```python
from build123d import *

# Parameters (mm, degrees)
SKETCH1_W           = 120
SKETCH1_H           = 150
SKETCH1_W_2         = 30
SKETCH1_H_2         = 50
BOSS_EXTRUDE1_DEPTH = 5


with BuildPart() as part:
    # Sketch1 → Boss-Extrude1 (new body)
    with BuildSketch(Plane.XY):
        Rectangle(SKETCH1_W, SKETCH1_H)
        with Locations((0, 35)):
            Rectangle(SKETCH1_W_2, SKETCH1_H_2, mode=Mode.SUBTRACT)
    extrude(amount=-BOSS_EXTRUDE1_DEPTH)


solid = part.part
```
Build history of the part. All positions in model axes, mm. A direction names the side the tool comes from. Give positions to 0.01 mm unless a question says otherwise; leave off trailing zeros. Loops run counter-clockwise (first coordinate to the right, second up) from the corner with the lowest first, then second, coordinate; pieces in that order, holes last.
1) Two-plate mould, pull along X, no slides. Class faces 1 (the face through (-1, 1, -5)), 2 (the face through (60, -1, -2)), 3 (the face through (-15, 35, -2)): released by +X, released by -X, zero draft, split by the parting line, or undercut.
Values follow:
face 1: zero draft
face 2: released by +X
face 3: undercut
2) Probe line 1 along X through (y, z) = (10.5, -0.4); line 2 along Y through (x, z) = (-10.5, -3.8). List the from-to ranges inside material, lowest first.
Values follow:
line 1: x = -60 to -15, 15 to 60
line 2: y = -75 to 10, 60 to 75
3) 3-axis set-ups, long thin cutter, end or side, ignore diameter. For faces 4 (the face through (-1, 1, 0)), 5 (the face through (0, 60, -2)): which of +Z, -Z, +X, -X, +Y, -Y reach the whole face in a straight line?
Values follow:
face 4: +Z, +X, -X, +Y, -Y
face 5: +Z, -Z
4) Band-saw the part on B-B on z = -3. List the corners of the cut face in (x, y), then the cut area to 3 significant figures.
Values follow:
outline: (-60, -75) - (60, -75) - (60, 75) - (-60, 75) - close; hole (-15, 10) - (15, 10) - (15, 60) - (-15, 60) - close
area: 16,500 mm2
5) Band-saw the part on A-A on y = 16. List the corners of the cut face in (x, z).
Values follow:
outline: (-60, -5) - (-15, -5) - (-15, 0) - (-60, 0) - close; (15, -5) - (60, -5) - (60, 0) - (15, 0) - close
6) Band-saw the part on C-C on x = 7.5. List the corners of the cut face in (y, z).
Values follow:
outline: (-75, -5) - (10, -5) - (10, 0) - (-75, 0) - close; (60, -5) - (75, -5) - (75, 0) - (60, 0) - close
